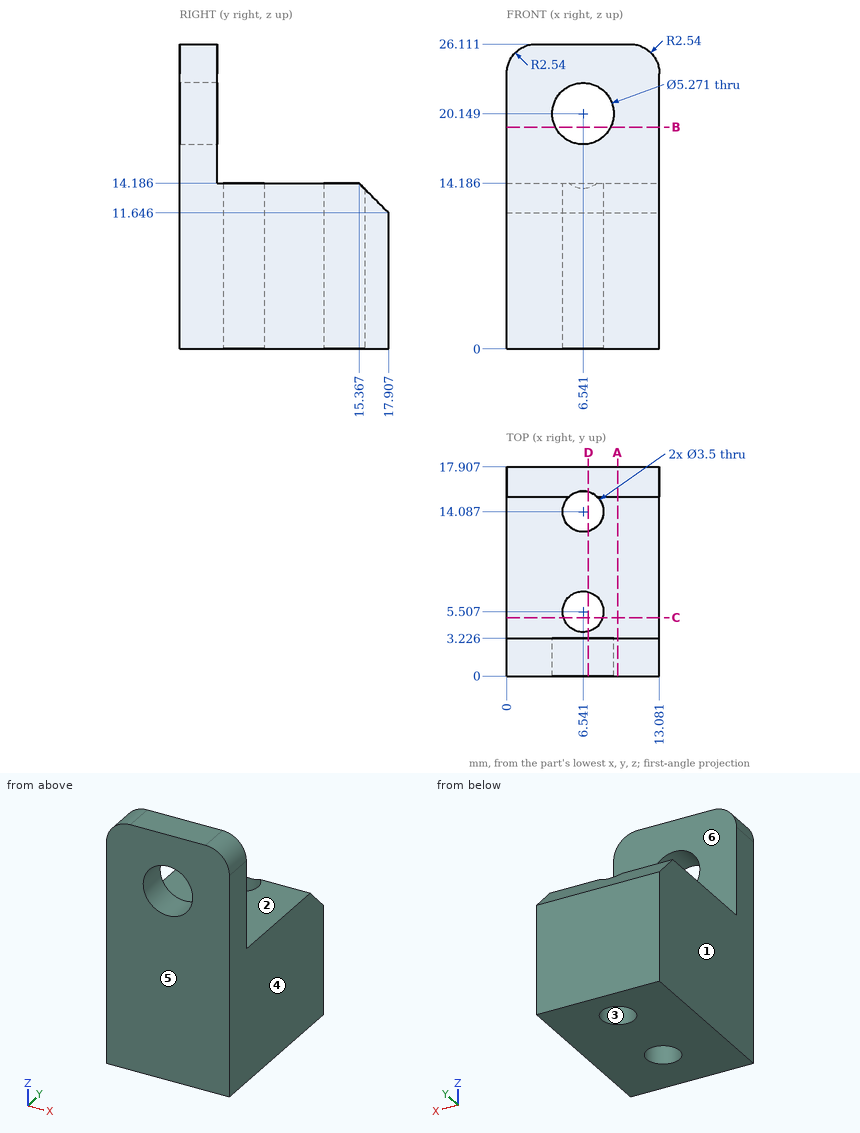
Geometry check sheet. Reference: drawing and pictorial views, mm from the part's lowest x, y, z. A direction names the side the tool comes from. Give positions to 0.01 mm unless a question says otherwise; leave off trailing zeros. Write each loop counter-clockwise with the first axis right and the second up, starting at its lowest first coordinate (ties: lowest second). Pieces come first, ordered by that corner, then holes. Notation, with made-up numbers: M 62.25,15.25 L 75.25,15.25 A18 ccw 75.25,40.25 Z; hole C 78.25,44.25 d7. An arc over 180 degrees is marked long. Put each result on its own line as item: value. Start each with the question number.
1. Section check D-D (x = 7). Record the cut outline in (y, z) (1 decimal), and give its area (3 significant figures).
2. Section check A-A (x = 9.5). Record the cut outline in (y, z) (1 decimal).
3. Scan lines: line 1 along Z through (x, y) = (12.5, 13.25) (1 decimal); line 2 along Y through (x, z) = (5.5, 15) (1 decimal); line 3 along Z through (x, y) = (5.5, 1). Record each from-to range of solid material in increasing order. Write a range as [from, to].
4. Go/stop test with flat-tipped pins: pin 1 Ø3 at (x, y) = (6.54, 5.51) entering from +Z; pin 2 Ø3.5 at (x, z) = (8.5, 17.5) entering from +Y; pin 3 Ø4.5 at (x, y) = (6.54, 14.09) entering from +Z. Record where each tip stops, or that it passes through.
5. Draft check along Y on the marked faces 3, 4, 5 and 6. Enter one of: +Y half, -Y half, draft (parallel to the pull), parting line (faces both ways), or undercut.
6. Section check B-B (z = 19). Record the cut outline in (x, y) (1 decimal), and give its area (3 significant figures).
7. Section check C-C (y = 5). Record the cut outline in (x, z) (1 decimal), and give its area (3 significant figures).
8. Set-up check for the marked faces 1 and 2: record each of +Z, -Z, +X, -X, +Y, -Y from which the full face is reachable in a straight line by a thin tool's end or side.
Answer list:
1. outline: M 0,0 L 3.8,0 L 3.8,14.2 L 3.2,14.2 L 3.2,17.6 L 0,17.6 Z; M 0,22.7 L 3.2,22.7 L 3.2,26.1 L 0,26.1 Z; M 7.2,0 L 12.4,0 L 12.4,14.2 L 7.2,14.2 Z; M 15.8,0 L 17.9,0 L 17.9,11.6 L 15.8,13.8 Z
1. area: 177 mm2
2. outline: M 0,0 L 17.9,0 L 17.9,11.6 L 15.4,14.2 L 3.2,14.2 L 3.2,26.1 L 0,26.1 Z
3. line 1: [0, 14.2]
3. line 2: [0, 3.2]
3. line 3: [0, 17.73], [22.57, 26.11]
4. pin 1: through
4. pin 2: y = 3.23
4. pin 3: z = 14.19
5. face 3: undercut
5. face 4: draft
5. face 5: -Y half
5. face 6: +Y half
6. outline: M 0,0 L 4.2,0 L 4.2,3.2 L 0,3.2 Z; M 8.9,0 L 13.1,0 L 13.1,3.2 L 8.9,3.2 Z
6. area: 26.9 mm2
7. outline: M 0,0 L 4.9,0 L 4.9,14.2 L 0,14.2 Z; M 8.2,0 L 13.1,0 L 13.1,14.2 L 8.2,14.2 Z
7. area: 138 mm2
8. face 1: +Z, -Z, -X, +Y, -Y
8. face 2: +Z, +X, -X, +Y
